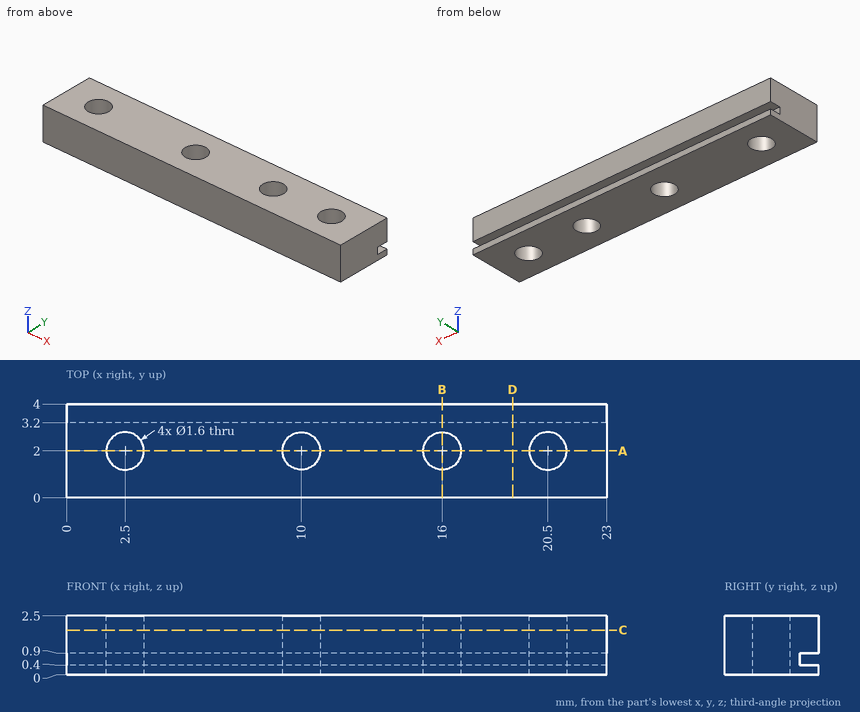
Check sheet for the drawn part. Datum: minimum x, y, z corner. Units: mm. Give positions to 0.01 mm unless a question says otherwise; leave off trailing zeros. Loops run counter-clockwise (first coordinate to the right, second up) from the corner with the lowest first, then second, coordinate; pieces in that order, holes last.
1) Sectioned sample at C-C, the plane z = 1.9. Enter the section's corners in (x, y).
2) Sectioned sample at A-A, the plane y = 2. Enter the section's corners in (x, z), then the cut area to 3 significant figures.
3) Sectioned sample at B-B, the plane x = 16. Enter the section's corners in (y, z), then the cut area to 3 significant figures.
4) Sectioned sample at D-D, the plane x = 19. Enter the section's corners in (y, z).
5) Depth check by flat-ended pin: pin 1 Ø1.5 at (x, y) = (3, 2) entering from -Z; pin 2 Ø1.4 at (x, y) = (20.5, 2) entering from -Z. Enter the tip coordinate at first touch or a pass-through.
6) Thickness scan on line 1 along Z through (x, y) = (19, 3.7); line 2 along Y through (x, z) = (20.5, 1.45); line 3 along X through (y, z) = (1.3, 2.35). Record the ranges inside material, lowest first.
Answers:
1. outline: (0, 0) - (23, 0) - (23, 4) - (0, 4) - close; hole circle Ø1.6 at (2.5, 2); hole circle Ø1.6 at (10, 2); hole circle Ø1.6 at (16, 2); hole circle Ø1.6 at (20.5, 2)
2. outline: (0, 0) - (1.7, 0) - (1.7, 2.5) - (0, 2.5) - close; (3.3, 0) - (9.2, 0) - (9.2, 2.5) - (3.3, 2.5) - close; (10.8, 0) - (15.2, 0) - (15.2, 2.5) - (10.8, 2.5) - close; (16.8, 0) - (19.7, 0) - (19.7, 2.5) - (16.8, 2.5) - close; (21.3, 0) - (23, 0) - (23, 2.5) - (21.3, 2.5) - close
2. area: 41.5 mm2
3. outline: (0, 0) - (1.2, 0) - (1.2, 2.5) - (0, 2.5) - close; (2.8, 0) - (4, 0) - (4, 0.4) - (3.2, 0.4) - (3.2, 0.9) - (4, 0.9) - (4, 2.5) - (2.8, 2.5) - close
3. area: 5.60 mm2
4. outline: (0, 0) - (4, 0) - (4, 0.4) - (3.2, 0.4) - (3.2, 0.9) - (4, 0.9) - (4, 2.5) - (0, 2.5) - close
5. pin 1: stops at z = 0
5. pin 2: passes through
6. line 1: z = 0 to 0.4, 0.9 to 2.5
6. line 2: y = 0 to 1.2, 2.8 to 4
6. line 3: x = 0 to 2.11, 2.89 to 9.61, 10.39 to 15.61, 16.39 to 20.11, 20.89 to 23
